The figure shows three views and two pictorial views of one solid part (mm, origin at its lowest corner). Answer the questions. Coordinates: 2 decimals unless noted, no trailing zeros. Loops run counter-clockwise (first coordinate to the right, second up) from the corner with the lowest first, then second, coordinate; pieces in that order, holes last. Notation, with made-up numbers: M 38,23.25 L 72,23.25 A6 ccw 72,34.25 Z; hole C 83.25,79.5 d5. An arc over 180 degrees is marked long. One line per item, written item: value. Start each with the question number.
1. The part is cut by section A-A (x = 40). Write down the section's boundary in (y, z), then the cut area to 3 significant figures.
2. The part is cut by section B-B (y = 2.2). State how many separate pieces and enclosed holes the cut face has, then the cut area to 3 significant figures.
3. The part is cut by section D-D (z = 75). Write down the section's boundary in (x, y).
4. A flat-ended cylindrical pin translates along its axis: pin 1 (5 mm diameter, centred on x = 30, z = 30, fed in from +Y). Find the tip coordinate at first contact, or state that the pin passes through.
5. The part is cut by section C-C (z = 40). Write down the section's boundary in (x, y), then the cut area to 3 significant figures.
6. Consider probe 1 along Z at (x, y) = (40, 1.45); probe 2 along X at (y, z) = (2.8, 47). Determine where each line is inside the solid, lowest interval first.
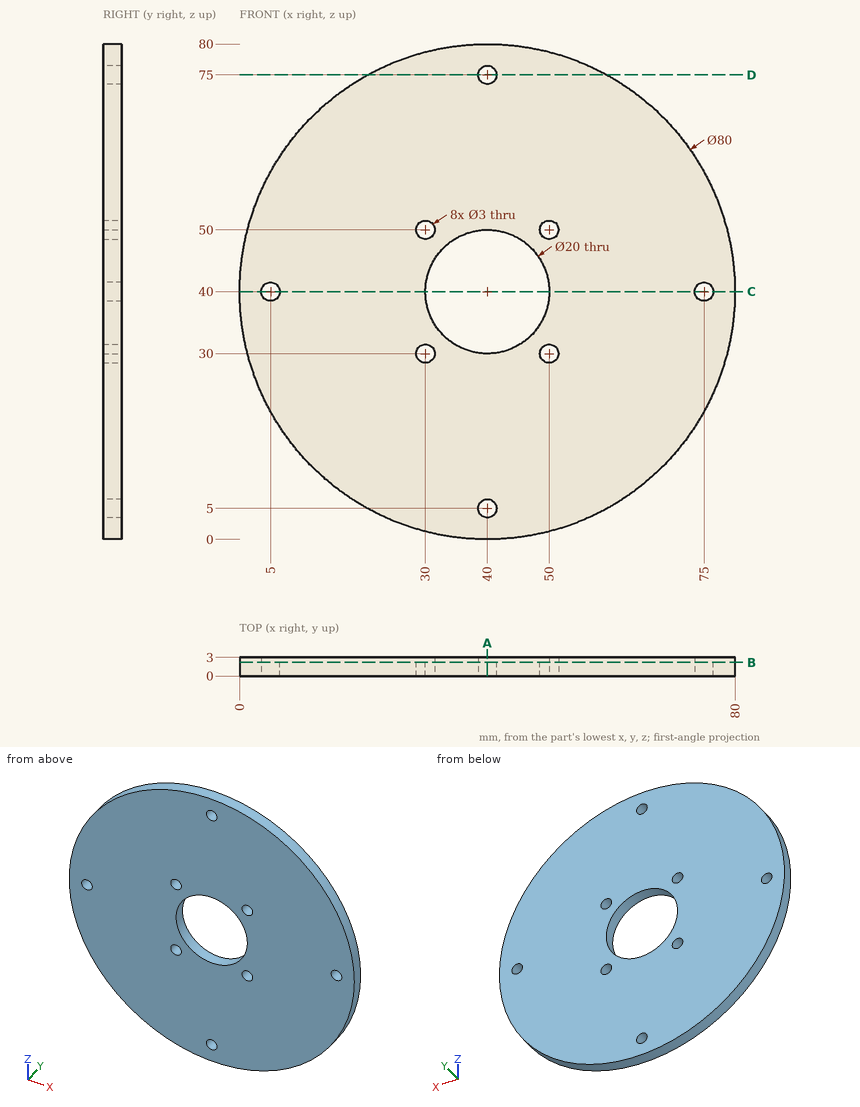
Answer block:
1. outline: M 0,0 L 3,0 L 3,3.5 L 0,3.5 Z; M 0,6.5 L 3,6.5 L 3,30 L 0,30 Z; M 0,50 L 3,50 L 3,73.5 L 0,73.5 Z; M 0,76.5 L 3,76.5 L 3,80 L 0,80 Z
1. area: 162 mm2
2. separate pieces: 1
2. enclosed holes: 9
2. area: 4,660 mm2
3. outline: M 20.64,0 L 38.5,0 L 38.5,3 L 20.64,3 Z; M 41.5,0 L 59.36,0 L 59.36,3 L 41.5,3 Z
4. pin 1: stops at y = 3
5. outline: M 0,0 L 3.5,0 L 3.5,3 L 0,3 Z; M 6.5,0 L 30,0 L 30,3 L 6.5,3 Z; M 50,0 L 73.5,0 L 73.5,3 L 50,3 Z; M 76.5,0 L 80,0 L 80,3 L 76.5,3 Z
5. area: 162 mm2
6. probe 1: z = 0 to 3.5, 6.5 to 30, 50 to 73.5, 76.5 to 80
6. probe 2: x = 0.62 to 32.86, 47.14 to 79.38
